from build123d import *

# Parameters (mm, degrees)
ESQUISSE2_W             = 151
ESQUISSE2_H             = 78
BOSS_EXTRU_1_DEPTH      = 23
ESQUISSE3_W             = 10
ESQUISSE3_H             = 2
ESQUISSE3_H_2           = 4.72
ENL_V_MAT_EXTRU_1_DEPTH = 7.31
CONG_1_R                = 11.2


with BuildPart() as part:
    # Esquisse2 → Boss.-Extru.1 (new body)
    with BuildSketch(Plane.XY):
        with Locations((-24.090850635, -9.469261584)):
            Rectangle(ESQUISSE2_W, ESQUISSE2_H)
    extrude(amount=BOSS_EXTRU_1_DEPTH)

    # Esquisse3 → Enlèv. mat.-Extru.1 (cut)
    with BuildSketch(Plane(origin=(51.409149365, 0, 0), x_dir=(0, 0, -1), z_dir=(1, 0, 0))):
        with Locations((-18, 5.630738416)):
            Rectangle(ESQUISSE3_W, ESQUISSE3_H)
        with Locations((-18, 10.630738416)):
            Rectangle(ESQUISSE3_W, ESQUISSE3_H)
        with Locations((-18, -12.169261584)):
            Rectangle(ESQUISSE3_W, ESQUISSE3_H_2)
        with Locations((-18, 15.630738416)):
            Rectangle(ESQUISSE3_W, ESQUISSE3_H)
        with Locations((-18, 0.630738416)):
            Rectangle(ESQUISSE3_W, ESQUISSE3_H)
        with Locations((-18, -4.369261584)):
            Rectangle(ESQUISSE3_W, ESQUISSE3_H)
    extrude(amount=-ENL_V_MAT_EXTRU_1_DEPTH, mode=Mode.SUBTRACT)

    # Congé1
    cong_1_edges = [part.edges().sort_by_distance(p)[0] for p in [
        (-24.090850635, 29.530738416, 23),
        (-24.090850635, 29.530738416, 0),
        (-24.090850635, -48.469261584, 0),
        (-24.090850635, -48.469261584, 23),
    ]]
    fillet(cong_1_edges, radius=CONG_1_R)


solid = part.part
Input: part model. Units: mm. Frame: model coordinates. A direction names the side the tool comes from. Give positions to 0.01 mm unless a question says otherwise; leave off trailing zeros. Write each loop counter-clockwise with the first axis right and the second up, starting at its lowest first coordinate (ties: lowest second). Pieces come first, ordered by that corner, then holes.
Q1. Set-up query: faces 1 (the face through (-23.03, -45.28, 19.63)), 2 (the face through (48, -5.369, 18)). Return all of +Z, -Z, +X, -X, +Y, -Y with unobstructed straight access to the full face (end or side cutting, diameter ignored); none if empty.
Q2. Section C-C, the plane z = 15.5. Output: boundary loops of the cut face in (x, y).
Q3. Section B-B, the plane y = -12. Output: boundary loops of the cut face in (x, z), plus the area to 3 significant figures.
Q4. Section A-A, the plane x = -88. Output: boundary loops of the cut face in (y, z).
Q5. First-contact query: P1, Ø2, axis at x = 46.5, z = 17, coming from the -Y side; P2, Ø8, axis at x = 46.5, z = 16, coming from the +Y side; P3, Ø2, axis at y = 10.5, z = 17, coming from the +X side; P4, Ø0.6, axis at y = 5.5, z = 19.5, coming from the +X side. Flat tips, straight axial feed; report the tip coordinate or a pass-through.
Q6. Material intervals for probe 1 along X at (y, z) = (16.5, 16.75); probe 2 along Z at (x, y) = (29, 21); probe 3 along Z at (x, y) = (2.5, 26.5), sorted ascending.
Q7. Pull-direction query (Y, two-part tool) for faces 3 (the face through (-23.03, -45.28, 3.37)), 4 (the face through (-25, -9, 0)), 5 (the face through (48, -0.369, 18)); classes: pulls with the +Y half, pulls with the -Y half, needs draft (parallel to the pull), parting line crosses it, or undercut.
Q8. Section D-D, the plane z = 5. Output: boundary loops of the cut face in (x, y).
Filled in:
1. face 1: +Z, +X, -X, -Y
1. face 2: +Z, +X
2. outline: (-99.59, -47.84) - (51.41, -47.84) - (51.41, -14.53) - (44.1, -14.53) - (44.1, -9.81) - (51.41, -9.81) - (51.41, -5.37) - (44.1, -5.37) - (44.1, -3.37) - (51.41, -3.37) - (51.41, -0.37) - (44.1, -0.37) - (44.1, 1.63) - (51.41, 1.63) - (51.41, 4.63) - (44.1, 4.63) - (44.1, 6.63) - (51.41, 6.63) - (51.41, 9.63) - (44.1, 9.63) - (44.1, 11.63) - (51.41, 11.63) - (51.41, 14.63) - (44.1, 14.63) - (44.1, 16.63) - (51.41, 16.63) - (51.41, 28.9) - (-99.59, 28.9) - close
3. outline: (-99.59, 0) - (51.41, 0) - (51.41, 13) - (44.1, 13) - (44.1, 23) - (-99.59, 23) - close
3. area: 3,400 mm2
4. outline: (-48.47, 11.2) arc R11.2 ccw to (-37.27, 0) - (18.33, 0) arc R11.2 ccw to (29.53, 11.2) - (29.53, 11.8) arc R11.2 ccw to (18.33, 23) - (-37.27, 23) arc R11.2 ccw to (-48.47, 11.8) - close
5. P1: stops at y = -47.65
5. P2: stops at y = 29.53
5. P3: stops at x = 51.41
5. P4: stops at x = 44.1
6. probe 1: x = -99.59 to 44.1
6. probe 2: z = 0.32 to 22.68
6. probe 3: z = 3.54 to 19.46
7. face 3: pulls with the -Y half
7. face 4: needs draft
7. face 5: undercut
8. outline: (-99.59, -46.6) - (51.41, -46.6) - (51.41, 27.66) - (-99.59, 27.66) - close
